from build123d import *

# Parameters (mm, degrees)
F0_R      = 15.4
F0_R_2    = 12.9
F1_DEPTH  = 20
F2_DEPTH  = 18.5
F3_R      = 4.1
F4_DEPTH  = 25
F6_DEPTH  = 20
F7_R      = 9.5
F7_R_2    = 5
F8_DEPTH  = 1.5
F9_DEPTH  = 20
F10_W     = 8.4
F10_H     = 20
F10_W_2   = 8.2
F11_DEPTH = 2
F12_R     = 1.5
F13_DEPTH = 3
F14_DEPTH = 1.25
F15_DEPTH = 1.25


with BuildPart() as f1:
    # F0 (on Top) → F1 (new body)
    with BuildSketch(Plane.XY):
        Circle(F0_R)
        Circle(F0_R_2, mode=Mode.SUBTRACT)
        Circle(F0_R_2)
    extrude(amount=F1_DEPTH)

    # F0 (on Top) → F2 (cut)
    with BuildSketch(Plane.XY):
        Circle(F0_R_2)
    extrude(amount=F2_DEPTH, mode=Mode.SUBTRACT)

    # F3 (on face) → F4 (cut)
    with BuildSketch(Plane.XY.offset(20)):
        Circle(F3_R)
    extrude(amount=-F4_DEPTH, mode=Mode.SUBTRACT)

    # F5 (on face) → F6 (join, through all)
    with BuildSketch(Plane.XY.offset(20)):
        with BuildLine():
            ThreePointArc((4.1, -14.8441907829), (0, -15.4), (-4.1, -14.8441907829))
            Line((-4.1, -14.8441907829), (-4.1, -138.7221455941))
            ThreePointArc((-4.1, -138.7221455941), (0, -138), (4.1, -138.7221455941))
            Line((4.1, -138.7221455941), (4.1, -14.8441907829))
        make_face()
        with BuildLine():
            ThreePointArc((4.1, -138.7221455941), (0, -138), (-4.1, -138.7221455941))
            Line((-4.1, -138.7221455941), (-4.1, -141.4302858857))
            ThreePointArc((-4.1, -141.4302858857), (0, -140.5), (4.1, -141.4302858857))
            Line((4.1, -141.4302858857), (4.1, -138.7221455941))
        make_face()
        with BuildLine():
            Line((-4.1, -141.4302858857), (-4.1, -138.7221455941))
            ThreePointArc((-4.1, -138.7221455941), (-6.8847657912, -159.8285299002), (12, -150))
            ThreePointArc((12, -150), (9.8285299002, -143.1152342088), (4.1, -138.7221455941))
            Line((4.1, -138.7221455941), (4.1, -141.4302858857))
            ThreePointArc((4.1, -141.4302858857), (8.037412519, -144.9354170952), (9.5, -150))
            ThreePointArc((9.5, -150), (-5.0645829048, -158.037412519), (-4.1, -141.4302858857))
        make_face()
    extrude(amount=-F6_DEPTH)

    # F7 (on face) → F8 (join, through all)
    with BuildSketch(Plane.XY.offset(20)):
        with Locations((0, -150)):
            Circle(F7_R)
        with Locations((0, -150)):
            Circle(F7_R_2, mode=Mode.SUBTRACT)
    extrude(amount=-F8_DEPTH)

    # F5 (on face) → F9 (join, through all)
    with BuildSketch(Plane.XY.offset(20)):
        with BuildLine():
            Line((-4.1, 20), (-4.1, 14.8441907829))
            ThreePointArc((-4.1, 14.8441907829), (0, 15.4), (4.1, 14.8441907829))
            Line((4.1, 14.8441907829), (4.1, 20))
            Line((4.1, 20), (-4.1, 20))
        make_face()
    extrude(amount=-F9_DEPTH)

    # F10 (on face) → F11 (join)
    with BuildSketch(Plane(origin=(0, 20, 0), x_dir=(-1, 0, 0), z_dir=(0, 1, 0))):
        with Locations((-8.3, 10)):
            Rectangle(F10_W, F10_H)
        with Locations((8.3, 10)):
            Rectangle(F10_W, F10_H)
        with Locations((0, 10)):
            Rectangle(F10_W_2, F10_H)
    extrude(amount=F11_DEPTH)

    # F12 (on face) → F13 (join)
    with BuildSketch(Plane(origin=(0, 22, 0), x_dir=(-1, 0, 0), z_dir=(0, 1, 0))):
        with Locations((-8.5, 18)):
            Circle(F12_R)
        with Locations((8.5, 18)):
            Circle(F12_R)
    extrude(amount=F13_DEPTH)

    # F14 (cut): a face of the model
    f14_faces = [f1.faces().sort_by_distance(p)[0] for p in [
        (12.5, 21, 10),
    ]]
    extrude(f14_faces, amount=-F14_DEPTH, mode=Mode.SUBTRACT)

    # F15 (cut): a face of the model
    f15_faces = [f1.faces().sort_by_distance(p)[0] for p in [
        (-12.5, 21, 10),
    ]]
    extrude(f15_faces, amount=-F15_DEPTH, mode=Mode.SUBTRACT)


solid = f1.part
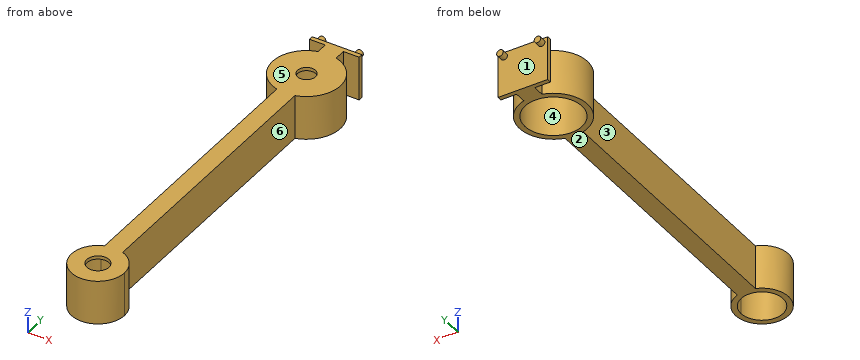
Part model, mm, in its own coordinate system. Face numbers are marked on the shaded views. A direction names the side the tool comes from. Coordinates: 2 decimals unless noted, no trailing zeros. Write each loop counter-clockwise with the first axis right and the second up, starting at its lowest first coordinate (ties: lowest second). Pieces come first, ordered by that corner, then holes. Notation, with made-up numbers: (3.5, -38) - (35.5, -38) arc R27 ccw to (35.5, -20) - close; hole circle Ø2 at (36, 33.25). An arc over 180 degrees is marked (long way). Put each result on its own line as item: value.
1. Probe line 1 along Y through (x, z) = (0, 19.65); line 2 along Y through (x, z) = (0, 4); line 3 along X through (y, z) = (-150, 10.5). List the from-to ranges inside material, lowest first. Write a range as [from, to].
Final values:
line 1: y = [-162, -155], [-145, -4.1], [4.1, 22]
line 2: y = [-162, -159.5], [-140.5, -12.9], [12.9, 22]
line 3: x = [-12, -9.5], [9.5, 12]
2. Two-plate mould, pull along Y, no slides. Class the marked faces 1, 2, 3 and 4: +Y half, -Y half, draft (parallel to the pull), parting line (faces both ways), or undercut.
Final values:
face 1: +Y half
face 2: draft
face 3: undercut
face 4: undercut
3. Band-saw the part on D-D (y = -49.5). Write the cut outline in (x, z), then the cut area to 3 significant figures.
Final values:
outline: (-4.1, 0) - (4.1, 0) - (4.1, 20) - (-4.1, 20) - close
area: 164 mm²
4. Band-saw the part on C-C (z = 13.75). Write the cut outline in (x, y), then the cut area to 3 significant figures.
Final values:
outline: (-11.25, 20) - (-4.1, 20) - (-4.1, 14.84) arc R15.4 ccw to (-4.1, -14.84) - (-4.1, -138.72) arc R12 ccw (long way) to (4.1, -138.72) - (4.1, -14.84) arc R15.4 ccw to (4.1, 14.84) - (4.1, 20) - (11.25, 20) - (11.25, 22) - (-11.25, 22) - close; hole circle Ø25.8 at (0, 0); hole circle Ø19 at (0, -150)
area: 1,480 mm²
5. Band-saw the part on B-B (y = 0). Write the cut outline in (x, z).
Final values:
outline: (-15.4, 0) - (-12.9, 0) - (-12.9, 18.5) - (-4.1, 18.5) - (-4.1, 20) - (-15.4, 20) - close; (4.1, 18.5) - (12.9, 18.5) - (12.9, 0) - (15.4, 0) - (15.4, 20) - (4.1, 20) - close
6. 3-axis set-ups, long thin cutter, end or side, ignore diameter. For the marked faces 5 and 6: which of +Z, -Z, +X, -X, +Y, -Y reach the whole face in a straight line?
Final values:
face 5: +Z, +X, -X, +Y, -Y
face 6: +Z, -Z, +X
7. Flat gauge pins, fed straight in: pin 1 Ø1 at (y, z) = (21.5, 5.5) entering from -X; pin 2 Ø5 at (y, z) = (4.5, 15.5) entering from -X; pin 3 Ø2.5 at (y, z) = (17, 14.5) entering from +X. Where does each tip first touch, or does it go through?
Final values:
pin 1: stops at x = -11.25
pin 2: stops at x = -15.27
pin 3: stops at x = 4.1
8. Band-saw the part on A-A (x = 0). Write the cut outline in (y, z), then the cut area to 3 significant figures.
Final values:
outline: (-162, 0) - (-159.5, 0) - (-159.5, 18.5) - (-155, 18.5) - (-155, 20) - (-162, 20) - close; (-145, 18.5) - (-140.5, 18.5) - (-140.5, 0) - (-12.9, 0) - (-12.9, 18.5) - (-4.1, 18.5) - (-4.1, 20) - (-145, 20) - close; (4.1, 18.5) - (12.9, 18.5) - (12.9, 0) - (22, 0) - (22, 20) - (4.1, 20) - close
area: 2,820 mm²
